Source: CAD feature listing. Evaluate the final solid. Frame: model axes, mm. Face numbers are marked on the shaded views. A direction names the side the tool comes from. Give positions to 0.01 mm unless a question says otherwise; leave off trailing zeros. Order: outer loops, then holes, each group sorted by start corner. A loop starts at its lowest first (then second) coordinate and runs counter-clockwise, first axis right, second up.
from build123d import *

# Parameters (mm, degrees)
BOSS_EXTRUDE1_DEPTH = 5
BOSS_EXTRUDE2_DEPTH = 40


with BuildPart() as part:
    # Sketch1 → Boss-Extrude1 (new body)
    with BuildSketch(Plane(origin=(0, 0, 0), x_dir=(1, 0, 0), z_dir=(0, 1, 0))):
        Polygon((10.55671577, 31.064383054), (-6.94328423, 31.064383054), (10.55671577, 6.210249778), align=None)
        Polygon((-6.94328423, 33.064383054), (-6.94328423, 31.064383054), (10.55671577, 31.064383054), (10.55671577, -31.935616946), (15.55671577, -31.935616946), (15.55671577, 33.064383054), align=None)
    extrude(amount=BOSS_EXTRUDE1_DEPTH)

    # Sketch1_3 → Boss-Extrude2 (add)
    with BuildSketch(Plane(origin=(0, 0, 0), x_dir=(1, 0, 0), z_dir=(0, 1, 0))):
        Polygon((-6.94328423, 33.064383054), (-6.94328423, 31.064383054), (10.55671577, 31.064383054), (10.55671577, -31.935616946), (15.55671577, -31.935616946), (15.55671577, 33.064383054), align=None)
    extrude(amount=-BOSS_EXTRUDE2_DEPTH)


solid = part.part
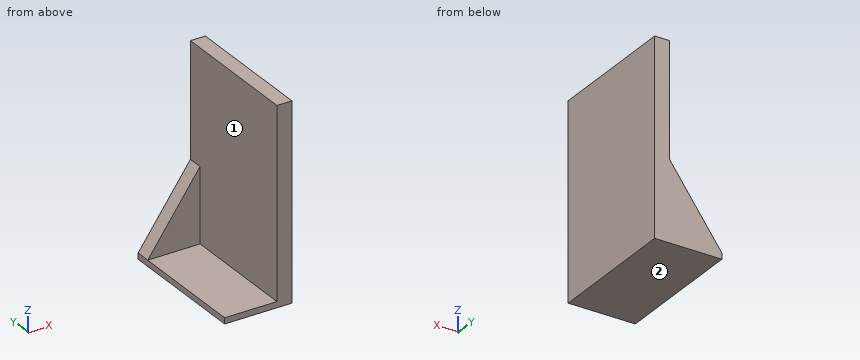
(1) Section A-A, the plane y = -12.5. Return loops of the section in (x, z).
(2) Section B-B, the plane x = 9.5. Return loops of the section in (y, z), plus the area to 3 significant figures.
(3) Section C-C, the plane z = -5. Return loops of the section in (x, y), plus the area to 3 significant figures.
(4) Line query: line 1 along Y through (x, z) = (1.5, -23.5); line 2 along X through (y, z) = (-15, 1.5); line 3 along Z through (x, y) = (4.75, -25.5). Output: solid intervals per line, ascending.
(5) Pin query (flat end, axial travel): pin 1 Ø5 at (y, z) = (-10.5, 5.5) entering from -X; pin 2 Ø5 at (x, z) = (-0.5, -14.5) entering from -Y; pin 3 Ø2 at (x, z) = (-2.5, -26.5) entering from -Y. Return the tip coordinate at first contact, or that it passes through.
(6) Access query for the marked faces 1 and 2. Directions: +Z, -Z, +X, -X, +Y, -Y. A direction counts if a zero-diameter tool reaches every point of the face in a straight line with its end or side. Return the directions, or none.
Checks:
1. outline: (-6.94, -33.06) - (15.56, -33.06) - (15.56, 31.94) - (10.56, 31.94) - (10.56, -31.06) - (-6.94, -31.06) - close
2. outline: (-40, -33.06) - (5, -33.06) - (5, -7.71) - (0, -7.71) - (0, -31.06) - (-40, -31.06) - close
2. area: 207 mm2
3. outline: (10.56, -40) - (15.56, -40) - (15.56, 5) - (10.56, 5) - close
3. area: 225 mm2
4. line 1: y = 0 to 5
4. line 2: x = 10.56 to 15.56
4. line 3: z = -33.06 to -31.06
5. pin 1: stops at x = 10.56
5. pin 2: passes through
5. pin 3: stops at y = 0
6. face 1: +Z, -X, -Y
6. face 2: -Z, +X, -X, +Y, -Y
